Model file for the job. Use its own axes, mm. Face numbers are marked on the shaded views. A direction names the side the tool comes from. Round coordinates to 2 decimals unless told otherwise and drop trailing zeros. Loops run counter-clockwise (first coordinate to the right, second up) from the corner with the lowest first, then second, coordinate; pieces in that order, holes last. Notation, with made-up numbers: M 0.5,16 L 14.5,16 A22 ccw 14.5,37 Z; hole C 16.25,-1.75 d1. An arc over 180 degrees is marked long. Use a Markdown table: item, result. Add a question column.
Q1. Cut at C-C (z = 13.5). Give the cut face in (x, y).
Q2. Tool access for the marked faces 4, 5, 6, 7 and 8: list every direction of +Z, -Z, +X, -X, +Y, -Y with a clear straight run to the whole face (end or side of a thin tool).
Q3. Cut at D-D (y = -4.75). Give the cut face in (x, z), plus the area to 3 significant figures.
Q4. Cut at A-A (x = 17). Give the cut face in (y, z) (3 decimals), plus the area to 3 significant figures.
Q5. Mould opens along Z. For the marked faces 1, 2 and 3 say: +Z half, -Z half, draft (parallel to the pull), parting line (faces both ways), or undercut.
Q6. Cut at B-B (x = 13). Give the cut face in (y, z) (3 decimals), plus the area to 3 significant figures.
Q7. Pin check, flat tips, straight feed: pin 1 (4.5 mm diameter, centred on x = 0.1, y = 9.86, fed in from -Z); pin 2 (14 mm diameter, centred on y = 5.5, z = 7.5, fed in from +X); pin 3 (4.5 mm diameter, centred on y = 5.47, z = 39.17, fed in from -X); pin 4 (0.6 mm diameter, centred on x = 7.5, z = 33.5, fed in from -Y). Stop position of each tip, or through.
Q8. Probe line 1 (Z direction, x = 4.5, y = 8.75); line 2 (Z direction, x = -1, y = -3.25); line 3 (Y direction, x = 3, z = 47). List the from-to ranges inside material, lowest first. Write a range as from..to.
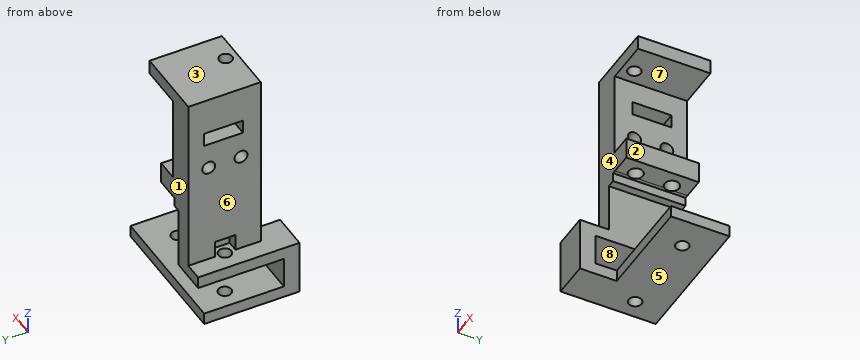
from build123d import *

# Parameters (mm, degrees)
SKETCH1_W                = 8
SKETCH1_H                = 24
SKETCH1_H_2              = 6
SKETCH1_H_3              = 26.58
SKETCH1_W_2              = 6
BOSS_EXTRUDE1_DEPTH      = 20
SKETCH2_W                = 0.38984803
SKETCH2_H                = 24.105830214
CUT_EXTRUDE1_DEPTH       = 20
SKETCH3_W                = 42.504801082
SKETCH3_H                = 61.271071749
CUT_EXTRUDE2_DEPTH       = 7
BOSS_EXTRUDE3_DEPTH      = 8
BOSS_EXTRUDE3_DEPTH_BACK = 20
SKETCH5_W                = 10
SKETCH5_H                = 3.373015501
SKETCH6_R                = 2
CUT_EXTRUDE3_DEPTH       = 6
SKETCH7_W                = 10
SKETCH7_H                = 4.325701587
BOSS_EXTRUDE4_DEPTH      = 12
SKETCH8_W                = 10
SKETCH8_H                = 3.285099304
BOSS_EXTRUDE5_DEPTH      = 22
SKETCH9_R                = 1.8
CUT_EXTRUDE4_DEPTH       = 20
SKETCH10_W               = 4.6581603
SKETCH10_H               = 5.7
CUT_EXTRUDE5_DEPTH       = 3
SKETCH12_R               = 1.8
CUT_EXTRUDE7_DEPTH       = 5
SKETCH13_R               = 1.8
CUT_EXTRUDE8_DEPTH       = 12
SKETCH14_W               = 3.285099304
SKETCH14_H               = 16.14069385
BOSS_EXTRUDE6_DEPTH      = 28
SKETCH15_R               = 1.8
CUT_EXTRUDE9_DEPTH       = 20
SKETCH16_W               = 1.97268601
SKETCH16_H               = 15.028302634
CUT_EXTRUDE10_DEPTH      = 2
SKETCH18_W               = 3.824807143
SKETCH18_H               = 10.692395384
CUT_EXTRUDE11_DEPTH      = 10


with BuildPart() as part:
    # Sketch1 → Boss-Extrude1 (new body)
    with BuildSketch(Plane(origin=(0, 0, 0), x_dir=(1, 0, 0), z_dir=(0, 1, 0))):
        with Locations((4, -44.58)):
            Rectangle(SKETCH1_W, SKETCH1_H)
        with Locations((4, -29.58)):
            Rectangle(SKETCH1_W, SKETCH1_H_2)
        with Locations((4, -13.29)):
            Rectangle(SKETCH1_W, SKETCH1_H_3)
        with Locations((11, -29.58)):
            Rectangle(SKETCH1_W_2, SKETCH1_H_2)
        Polygon((8, -56.58), (0, -56.58), (0, -60.58), (20, -60.58), (20, -56.58), align=None)
    extrude(amount=BOSS_EXTRUDE1_DEPTH)

    # Sketch2 → Cut-Extrude1 (cut)
    with BuildSketch(Plane(origin=(0, 0, 0), x_dir=(-1, 0, 0), z_dir=(0, -1, 0))):
        Polygon((-7.155800491, -26.605830214), (-7.155800491, -24.105830214), (-8, -24.105830214), (-8, -26.58), (-8.155800491, -26.58), (-8.155800491, -26.605830214), align=None)
        Polygon((-8, -24.105830214), (-7.155800491, -24.105830214), (-5.353625866, -24.105830214), (-5.353625866, 0), (-8, 0), align=None)
        with Locations((-5.158701851, -12.052915107)):
            Rectangle(SKETCH2_W, SKETCH2_H)
    extrude(amount=-CUT_EXTRUDE1_DEPTH, mode=Mode.SUBTRACT)

    # Sketch3 → Cut-Extrude2 (cut)
    with BuildSketch(Plane(origin=(0, 0, 0), x_dir=(-1, 0, 0), z_dir=(0, 0, -1))):
        with Locations((-1.640387793, 8.242348963)):
            Rectangle(SKETCH3_W, SKETCH3_H)
    extrude(amount=-CUT_EXTRUDE2_DEPTH, mode=Mode.SUBTRACT)

    # Sketch5 → Boss-Extrude3 (add, two sides: drawn at the far end of the back side and taken through both)
    with BuildSketch(Plane(origin=(0, 0, 0), x_dir=(-1, 0, 0), z_dir=(0, -1, 0)).offset(-BOSS_EXTRUDE3_DEPTH_BACK)):
        with Locations((0.036222164, -8.686507751)):
            Rectangle(SKETCH5_W, SKETCH5_H)
    extrude(amount=BOSS_EXTRUDE3_DEPTH + BOSS_EXTRUDE3_DEPTH_BACK)

    # Sketch6 → Cut-Extrude3 (cut)
    with BuildSketch(Plane(origin=(0, 0, 26.58), x_dir=(-1, 0, 0), z_dir=(0, 0, -1))):
        with Locations(Location((-9.655800491, 4.904630263, 0), (0, 0, 34.116357222))):
            Circle(SKETCH6_R)
        with Locations(Location((-9.655800491, 14.904630263, 0), (0, 0, 325.883642778))):
            Circle(SKETCH6_R)
    extrude(amount=-CUT_EXTRUDE3_DEPTH, mode=Mode.SUBTRACT)

    # Sketch7 → Boss-Extrude4 (add)
    with BuildSketch(Plane(origin=(0, 0, 7), x_dir=(-1, 0, 0), z_dir=(0, 0, -1))):
        with Locations((0.036222164, -5.837149207)):
            Rectangle(SKETCH7_W, SKETCH7_H)
    extrude(amount=BOSS_EXTRUDE4_DEPTH)

    # Sketch8 → Boss-Extrude5 (add)
    with BuildSketch(Plane(origin=(0, -3.674298413, 0), x_dir=(1, 0, 0), z_dir=(0, 1, 0))):
        with Locations((-0.036222164, 3.357450348)):
            Rectangle(SKETCH8_W, SKETCH8_H)
    extrude(amount=BOSS_EXTRUDE5_DEPTH)

    # Sketch9 → Cut-Extrude4 (cut)
    with BuildSketch(Plane(origin=(0, 0, -5), x_dir=(-1, 0, 0), z_dir=(0, 0, -1))):
        with Locations((-0.102745826, 9.860584284)):
            Circle(SKETCH9_R)
    extrude(amount=-CUT_EXTRUDE4_DEPTH, mode=Mode.SUBTRACT)

    # Sketch10 → Cut-Extrude5 (cut)
    with BuildSketch(Plane.ZY):
        with Locations((12.702095651, 9.85)):
            Rectangle(SKETCH10_W, SKETCH10_H)
    extrude(amount=-CUT_EXTRUDE5_DEPTH, mode=Mode.SUBTRACT)

    # Sketch12 → Cut-Extrude7 (cut)
    with BuildSketch(Plane.XY.offset(60.58)):
        with Locations((12, 3.26546718)):
            Circle(SKETCH12_R)
    extrude(amount=-CUT_EXTRUDE7_DEPTH, mode=Mode.SUBTRACT)

    # Sketch13 → Cut-Extrude8 (cut)
    with BuildSketch(Plane.ZY):
        with Locations((39.167156573, 5.468808009)):
            Circle(SKETCH13_R)
        with Locations((39.167156573, 14.370824603)):
            Circle(SKETCH13_R)
    extrude(amount=-CUT_EXTRUDE8_DEPTH, mode=Mode.SUBTRACT)

    # Sketch14 → Boss-Extrude6 (add)
    with BuildSketch(Plane(origin=(4.963777836, 0, 0), x_dir=(0, 0, -1), z_dir=(1, 0, 0))):
        with Locations((3.357450348, 10.255354662)):
            Rectangle(SKETCH14_W, SKETCH14_H)
    extrude(amount=BOSS_EXTRUDE6_DEPTH)

    # Sketch15 → Cut-Extrude9 (cut)
    with BuildSketch(Plane(origin=(0, 0, -5), x_dir=(-1, 0, 0), z_dir=(0, 0, -1))):
        with Locations((-24.353207193, 9.904630263)):
            Circle(SKETCH15_R)
    extrude(amount=-CUT_EXTRUDE9_DEPTH, mode=Mode.SUBTRACT)

    # Sketch16 → Cut-Extrude10 (cut)
    with BuildSketch(Plane(origin=(8, 0, 0), x_dir=(0, 0, -1), z_dir=(1, 0, 0))):
        with Locations((-33.566343005, 9.65070179)):
            Rectangle(SKETCH16_W, SKETCH16_H)
    extrude(amount=-CUT_EXTRUDE10_DEPTH, mode=Mode.SUBTRACT)

    # Sketch18 → Cut-Extrude11 (cut)
    with BuildSketch(Plane.ZY):
        with Locations((48.45250386, 10.297450391)):
            Rectangle(SKETCH18_W, SKETCH18_H)
    extrude(amount=-CUT_EXTRUDE11_DEPTH, mode=Mode.SUBTRACT)


solid = part.part
Checked values:
| question | item | result |
|---|---|---|
| 1 | outline | M 0,0 L 4.96,0 L 4.96,20 L 0,20 L 0,12.7 L 3,12.7 L 3,7 L 0,7 Z |
| 2 | face 4 | +Z, +X, -X, -Y |
| 2 | face 5 | -Z, +X, -X, +Y, -Y |
| 2 | face 6 | +Z, -X, +Y, -Y |
| 2 | face 7 | +X, +Y, -Y |
| 2 | face 8 | +X, -X, +Y |
| 3 | outline | M -5.04,-5 L 4.96,-5 L 4.96,10.37 L -5.04,10.37 Z |
| 3 | area | 154 mm^2 |
| 4 | outline | M 0,56.58 L 20,56.58 L 20,60.58 L 0,60.58 Z; M 2.185,-5 L 18.326,-5 L 18.326,-1.715 L 2.185,-1.715 Z |
| 4 | area | 133 mm^2 |
| 5 | face 1 | draft |
| 5 | face 2 | undercut |
| 5 | face 3 | +Z half |
| 6 | outline | M 0,26.58 L 20,26.58 L 20,32.58 L 0,32.58 Z; M 0,56.58 L 1.769,56.58 L 1.769,60.58 L 0,60.58 Z; M 2.185,-5 L 18.326,-5 L 18.326,-1.715 L 2.185,-1.715 Z; M 4.762,56.58 L 20,56.58 L 20,60.58 L 4.762,60.58 Z |
| 6 | area | 241 mm^2 |
| 7 | pin 1 | stops at z = -5 |
| 7 | pin 2 | stops at x = 4.96 |
| 7 | pin 3 | stops at x = 0 |
| 7 | pin 4 | stops at y = 0 |
| 8 | line 1 | z = -5..-1.71, 7..46.54, 50.36..60.58 |
| 8 | line 2 | z = -5..-1.71, 7..10.37 |
| 8 | line 3 | y = 0..4.95, 15.64..20 |
